```python
from build123d import *

# Parameters (mm, degrees)
EXTRUDE_1_DEPTH     = 214.5
EXTRUDE_2_DEPTH     = 2
EXTRUDE_START       = 2
EXTRUDE_3_DEPTH     = 2
FILLET_2_R          = 3
FILLET_3_R          = 3
SKETCH_6_W          = 40
SKETCH_6_H          = 12
SKETCH_6_R          = 1.6
SKETCH_6_W_2        = 13
SKETCH_6_H_2        = 40
EXTRUDE_4_DEPTH     = 2
SKETCH_8_W          = 31
SKETCH_8_H          = 14
CUT_EXTRUDE_2_DEPTH = 10
FILLET_4_R          = 2
FILLET_5_R          = 2
SKETCH_9_W          = 42
SKETCH_9_H          = 50
CUT_EXTRUDE_3_DEPTH = 273.635746006
SKETCH_10_W         = 42
SKETCH_10_H         = 50
CUT_EXTRUDE_4_DEPTH = 273.635746006


with BuildPart() as part:
    # 草图1 → 凸台-拉伸1 (new body)
    with BuildSketch(Plane.XY):
        with BuildLine():
            Line((-68, 0), (64, 0))
            ThreePointArc((64, 0), (68.242640687, 1.757359313), (70, 6))
            Line((70, 6), (70, 53))
            Line((70, 53), (68, 53))
            Line((68, 53), (68, 7))
            ThreePointArc((68, 7), (66.535533906, 3.464466094), (63, 2))
            Line((63, 2), (-67, 2))
            ThreePointArc((-67, 2), (-70.535533906, 3.464466094), (-72, 7))
            Line((-72, 7), (-72, 53))
            Line((-72, 53), (-74, 53))
            Line((-74, 53), (-74, 6))
            ThreePointArc((-74, 6), (-72.242640687, 1.757359313), (-68, 0))
        make_face()
    extrude(amount=EXTRUDE_1_DEPTH)

    # 草图2 → 凸台-拉伸2 (add)
    with BuildSketch(Plane.XY.offset(214.5)):
        with BuildLine():
            Line((-68, 0), (64, 0))
            ThreePointArc((64, 0), (68.242640687, 1.757359313), (70, 6))
            Line((70, 6), (70, 53))
            Line((70, 53), (-74, 53))
            Line((-74, 53), (-74, 6))
            ThreePointArc((-74, 6), (-72.242640687, 1.757359313), (-68, 0))
        make_face()
    extrude(amount=EXTRUDE_2_DEPTH)

    # 草图3 → 凸台-拉伸3 (add)
    with BuildSketch(Plane(origin=(0, 0, 0), x_dir=(-1, 0, 0), z_dir=(0, 0, -1)).offset(EXTRUDE_START)):
        with BuildLine():
            Line((-64, 0), (68, 0))
            ThreePointArc((68, 0), (72.242640687, 1.757359313), (74, 6))
            Line((74, 6), (74, 53))
            Line((74, 53), (-70, 53))
            Line((-70, 53), (-70, 6))
            ThreePointArc((-70, 6), (-68.242640687, 1.757359313), (-64, 0))
        make_face()
    extrude(amount=-EXTRUDE_3_DEPTH)

    # 圆角2
    fillet_2_edges = [part.edges().sort_by_distance(p)[0] for p in [
        (68, 30, 214.5),
        (66.535533906, 3.464466094, 214.5),
        (-2, 2, 214.5),
        (-70.535533906, 3.464466094, 214.5),
        (-72, 30, 214.5),
    ]]
    fillet(fillet_2_edges, radius=FILLET_2_R)

    # 圆角3
    fillet_3_edges = [part.edges().sort_by_distance(p)[0] for p in [
        (-72, 30, 0),
        (-70.535533906, 3.464466094, 0),
        (-2, 2, 0),
        (66.535533906, 3.464466094, 0),
        (68, 30, 0),
    ]]
    fillet(fillet_3_edges, radius=FILLET_3_R)

    # 草图6 → 凸台-拉伸4 (add)
    # profile 1 of 4: a face of its own
    with BuildSketch(Plane(origin=(0, 53, 0), x_dir=(1, 0, 0), z_dir=(0, 1, 0))):
        with Locations((-36, 8)):
            Rectangle(SKETCH_6_W, SKETCH_6_H)
        with Locations(Location((-46, 10, 0), (0, 0, 270))):
            Circle(SKETCH_6_R, mode=Mode.SUBTRACT)
        with Locations(Location((-26, 10, 0), (0, 0, 270))):
            Circle(SKETCH_6_R, mode=Mode.SUBTRACT)
    # profile 2 of 4: a face of its own
    with BuildSketch(Plane(origin=(0, 53, 0), x_dir=(1, 0, 0), z_dir=(0, 1, 0))):
        with Locations((-80.5, -118)):
            Rectangle(SKETCH_6_W_2, SKETCH_6_H_2)
        with Locations(Location((-83, -108, 0), (0, 0, 270))):
            Circle(SKETCH_6_R, mode=Mode.SUBTRACT)
        with Locations(Location((-83, -128, 0), (0, 0, 270))):
            Circle(SKETCH_6_R, mode=Mode.SUBTRACT)
    # profile 3 of 4: a face of its own
    with BuildSketch(Plane(origin=(0, 53, 0), x_dir=(1, 0, 0), z_dir=(0, 1, 0))):
        with Locations((76.5, -118)):
            Rectangle(SKETCH_6_W_2, SKETCH_6_H_2)
        with Locations(Location((79, -128, 0), (0, 0, 90))):
            Circle(SKETCH_6_R, mode=Mode.SUBTRACT)
        with Locations(Location((79, -108, 0), (0, 0, 90))):
            Circle(SKETCH_6_R, mode=Mode.SUBTRACT)
    # profile 4 of 4: a face of its own
    with BuildSketch(Plane(origin=(0, 53, 0), x_dir=(1, 0, 0), z_dir=(0, 1, 0))):
        with Locations((32, 8)):
            Rectangle(SKETCH_6_W, SKETCH_6_H)
        with Locations(Location((42, 10, 0), (0, 0, 90))):
            Circle(SKETCH_6_R, mode=Mode.SUBTRACT)
        with Locations(Location((22, 10, 0), (0, 0, 90))):
            Circle(SKETCH_6_R, mode=Mode.SUBTRACT)
    extrude(amount=-EXTRUDE_4_DEPTH)

    # 草图8 → 切除-拉伸2 (cut)
    with BuildSketch(Plane.XY.offset(216.5)):
        with Locations((8.5, 46)):
            Rectangle(SKETCH_8_W, SKETCH_8_H)
    extrude(amount=-CUT_EXTRUDE_2_DEPTH, mode=Mode.SUBTRACT)

    # 圆角4
    fillet_4_edges = [part.edges().sort_by_distance(p)[0] for p in [
        (-36, 51, -2),
        (32, 51, -2),
        (-74, 51, 118),
        (70, 51, 118),
    ]]
    fillet(fillet_4_edges, radius=FILLET_4_R)

    # 圆角5
    fillet_5_edges = [part.edges().sort_by_distance(p)[0] for p in [
        (70, 29.5, 216.5),
        (-74, 29.5, 216.5),
        (-72.242640687, 1.757359313, 216.5),
        (-2, 0, 216.5),
        (68.242640687, 1.757359313, 216.5),
        (-74, 29.5, -2),
        (70, 29.5, -2),
        (68.242640687, 1.757359313, -2),
        (-2, 0, -2),
        (-72.242640687, 1.757359313, -2),
    ]]
    fillet(fillet_5_edges, radius=FILLET_5_R)

    # 草图9 → 切除-拉伸3 (cut, through all)
    with BuildSketch(Plane(origin=(70, 0, 0), x_dir=(0, 0, -1), z_dir=(1, 0, 0))):
        with Locations((-181.5, 28)):
            Rectangle(SKETCH_9_W, SKETCH_9_H)
    extrude(amount=-CUT_EXTRUDE_3_DEPTH, mode=Mode.SUBTRACT)

    # 草图10 → 切除-拉伸4 (cut, through all)
    with BuildSketch(Plane(origin=(70, 0, 0), x_dir=(0, 0, -1), z_dir=(1, 0, 0))):
        with Locations((-33, 28)):
            Rectangle(SKETCH_10_W, SKETCH_10_H)
    extrude(amount=-CUT_EXTRUDE_4_DEPTH, mode=Mode.SUBTRACT)


solid = part.part
```
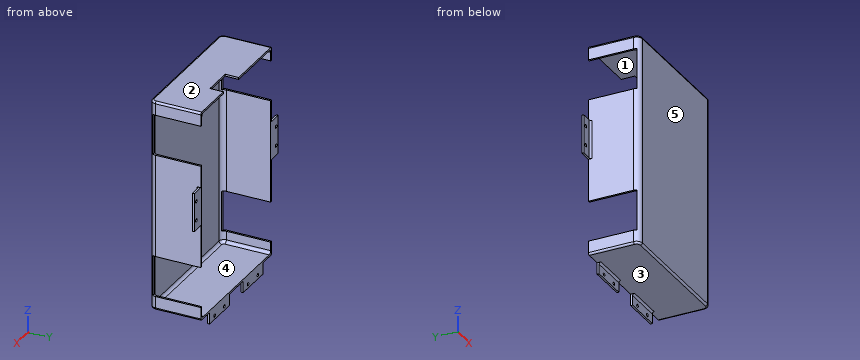
Design review of the part built by this model. Coordinates are the model's own, in mm. Face numbers are marked on the shaded views. A direction names the side the tool comes from. Round coordinates to 2 decimals unless told otherwise and drop trailing zeros. Order: outer loops, then holes, each group sorted by start corner. A loop starts at its lowest first (then second) coordinate and runs counter-clockwise, first axis right, second up. Notation, with made-up numbers: M 69.25,7.5 L 112.25,7.5 A18 cw 112.25,27.5 Z; hole C 54,-37.75 d9. An arc over 180 degrees is marked long. Put each result on its own line as item: value.
Q1. Consider section C-C (z = 49). State the section outline as (x, y) points.
Reported:
outline: M -73.2,3 A6 ccw -68,0 L 64,0 A6 ccw 69.2,3 L 66,3 A5 cw 63,2 L -67,2 A5 cw -70,3 Z
Q2. Insertion check: pin 1 Ø3 at (y, z) = (50, -8) entering from -X; pin 2 Ø2 at (y, z) = (34.5, 87.5) entering from +X; pin 3 Ø2 at (x, y) = (68, 24.5) entering from -Z; pin 4 Ø24 at (x, y) = (-4.5, 40.5) entering from +Z. Each pin has a flat end and moves straight along its axis. Give the tip position at first contact, or say it passes through.
Reported:
pin 1: x = -56
pin 2: x = 70
pin 3: z = -2
pin 4: z = 216.5
Q3. Consider section B-B (y = 26). State how many separate pieces and enclosed holes the cut face has, and give its area (3 significant figures).
Reported:
separate pieces: 4
enclosed holes: 0
area: 1,100 mm²
Q4. Machinability: for the marked faces 4 and 5, which of the approach directions +Z, -Z, +X, -X, +Y, -Y give a long, thin tool a straight path to every point of the face, cutting with its end or side? Answer none if there is none.
Reported:
face 4: +Y
face 5: +Z, -Z, +X, -X, -Y
Q5. Consider section A-A (x = -1.5). State the section outline as (y, z) points.
Reported:
outline: M 0,0 A2 ccw 2,-2 L 53,-2 L 53,0 L 5,0 A3 cw 2,3 L 2,211.5 A3 cw 5,214.5 L 39,214.5 L 39,216.5 L 2,216.5 A2 ccw 0,214.5 Z
Q6. Draft analysis for pull direction Z (two halves, no side actions). For the marked faces 1, 2 and 3, state which applies: released by +Z, released by -Z, zero draft, split by the parting line, or undercut.
Reported:
face 1: undercut
face 2: released by +Z
face 3: released by -Z
Q7. Consider section D-D (x = 30.5). State the section outline as (y, z) points, and give its area (3 significant figures).
Reported:
outline: M 0,0 A2 ccw 2,-2 L 49,-2 A2 cw 51,-4 L 51,-14 L 53,-14 L 53,0 L 5,0 A3 cw 2,3 L 2,211.5 A3 cw 5,214.5 L 53,214.5 L 53,216.5 L 2,216.5 A2 ccw 0,214.5 Z
area: 668 mm²
Q8. To check wall thickness, follow line 1 (Z direction, x = -83, y = 51.5); line 2 (X direction, y = 52.6, z = -10); line 3 (Z direction, x = 59, y = 9). State the ranges of each line that lie inside material, in increasing order.
Reported:
line 1: 98 to 106.4, 109.6 to 126.4, 129.6 to 138
line 2: -56 to -47.6, -44.4 to -27.6, -24.4 to -16, 12 to 20.4, 23.6 to 40.4, 43.6 to 52
line 3: -2 to 0, 214.5 to 216.5
